```python
from build123d import *

# Parameters (mm, degrees)
BOSS_EXTRUDE1_DEPTH  = 90
BOSS_EXTRUDE2_DEPTH  = 70
BOSS_EXTRUDE4_DEPTH  = 10
SKETCH4_W            = 20
SKETCH4_H            = 40
BOSS_EXTRUDE6_DEPTH  = 20
CUT_EXTRUDE1_DEPTH   = 20
SKETCH9_W            = 20
SKETCH9_H            = 20
BOSS_EXTRUDE8_DEPTH  = 10
SKETCH10_W           = 20
SKETCH10_H           = 10
CUT_EXTRUDE2_DEPTH   = 10
BOSS_EXTRUDE9_START  = -10
BOSS_EXTRUDE9_DEPTH  = 20
SKETCH13_W           = 26.1880454
SKETCH13_H           = 20
BOSS_EXTRUDE13_DEPTH = 30
CUT_EXTRUDE3_DEPTH   = 10
BOSS_EXTRUDE14_DEPTH = 30
BOSS_EXTRUDE15_DEPTH = 30
BOSS_EXTRUDE16_DEPTH = 40
BOSS_EXTRUDE17_DEPTH = 40
BOSS_EXTRUDE18_DEPTH = 10


with BuildPart() as part:
    # Sketch1 → Boss-Extrude1 (new body)
    with BuildSketch(Plane.XY):
        Polygon((0, 0), (0, 30), (40, 30), (40, -30), (20, -30), (20, -20), align=None)
    extrude(amount=BOSS_EXTRUDE1_DEPTH)

    # Sketch2 → Boss-Extrude2 (add)
    with BuildSketch(Plane.XY.offset(70)):
        Polygon((0, 30), (-30, 30), (-30, 20), (-20, 20), (0, 0), align=None)
    extrude(amount=-BOSS_EXTRUDE2_DEPTH)

    # Sketch3 → Boss-Extrude4 (add)
    with BuildSketch(Plane(origin=(0, 30, 0), x_dir=(1, 0, 0), z_dir=(0, 1, 0))):
        Polygon((-30, -60), (-50, -40), (-30, -40), align=None)
    extrude(amount=-BOSS_EXTRUDE4_DEPTH)

    # Sketch4 → Boss-Extrude6 (add)
    with BuildSketch(Plane(origin=(0, 30, 0), x_dir=(1, 0, 0), z_dir=(0, 1, 0))):
        with Locations((-40, -20)):
            Rectangle(SKETCH4_W, SKETCH4_H)
    extrude(amount=-BOSS_EXTRUDE6_DEPTH)

    # Sketch6 → Cut-Extrude1 (cut)
    with BuildSketch(Plane.ZY.offset(50)):
        Polygon((40, 20), (30, 10), (40, 10), align=None)
    extrude(amount=-CUT_EXTRUDE1_DEPTH, mode=Mode.SUBTRACT)

    # Sketch9 → Boss-Extrude8 (add)
    with BuildSketch(Plane.XZ.offset(-10)):
        with Locations((-40, 10)):
            Rectangle(SKETCH9_W, SKETCH9_H)
    extrude(amount=BOSS_EXTRUDE8_DEPTH)

    # Sketch10 → Cut-Extrude2 (cut)
    with BuildSketch(Plane.ZY.offset(50)):
        with Locations((10, 5)):
            Rectangle(SKETCH10_W, SKETCH10_H)
    extrude(amount=-CUT_EXTRUDE2_DEPTH, mode=Mode.SUBTRACT)

    # Sketch11 → Boss-Extrude9 (add)
    with BuildSketch(Plane(origin=(-30, 0, 0), x_dir=(0, 0, -1), z_dir=(1, 0, 0)).offset(BOSS_EXTRUDE9_START)):
        Polygon((-20, 0), (-30, 10), (-20, 10), align=None)
    extrude(amount=BOSS_EXTRUDE9_DEPTH)

    # Sketch13 → Boss-Extrude13 (add)
    with BuildSketch(Plane(origin=(0, 0, 0), x_dir=(-1, 0, 0), z_dir=(0, 0, -1))):
        with Locations((16.9059773, 10)):
            Rectangle(SKETCH13_W, SKETCH13_H)
    extrude(amount=-BOSS_EXTRUDE13_DEPTH)

    # Sketch14 → Cut-Extrude3 (cut)
    with BuildSketch(Plane.ZY.offset(30)):
        Polygon((20, 0), (30, 10), (30, 0), align=None)
    extrude(amount=-CUT_EXTRUDE3_DEPTH, mode=Mode.SUBTRACT)

    # Sketch15 → Boss-Extrude14 (add)
    with BuildSketch(Plane.ZY.offset(50)):
        Polygon((30, 10), (30, 20), (40, 20), align=None)
    extrude(amount=-BOSS_EXTRUDE14_DEPTH)

    # Sketch16 → Boss-Extrude15 (add)
    with BuildSketch(Plane.XZ.offset(30)):
        Polygon((20, 0), (10, 0), (10, 40), (20, 60), align=None)
    extrude(amount=-BOSS_EXTRUDE15_DEPTH)

    # Sketch17 → Boss-Extrude16 (add)
    with BuildSketch(Plane(origin=(0, 0, 0), x_dir=(-1, 0, 0), z_dir=(0, 0, -1))):
        Polygon((-10, -30), (20, -10), (20, 0), (0, 0), (-10, -10), align=None)
    extrude(amount=-BOSS_EXTRUDE16_DEPTH)

    # Sketch18 → Boss-Extrude17 (add)
    with BuildSketch(Plane(origin=(0, 0, 0), x_dir=(-1, 0, 0), z_dir=(0, 0, -1))):
        Polygon((3.8119546, 3.8119546), (3.8119546, 0), (0, 0), align=None)
    extrude(amount=-BOSS_EXTRUDE17_DEPTH)

    # Sketch19 → Boss-Extrude18 (add)
    with BuildSketch(Plane.XY.offset(30)):
        Polygon((-3.8119546, 3.8119546), (-3.8119546, 0), (-20, 0), (-20, 20), align=None)
    extrude(amount=BOSS_EXTRUDE18_DEPTH)


solid = part.part
```
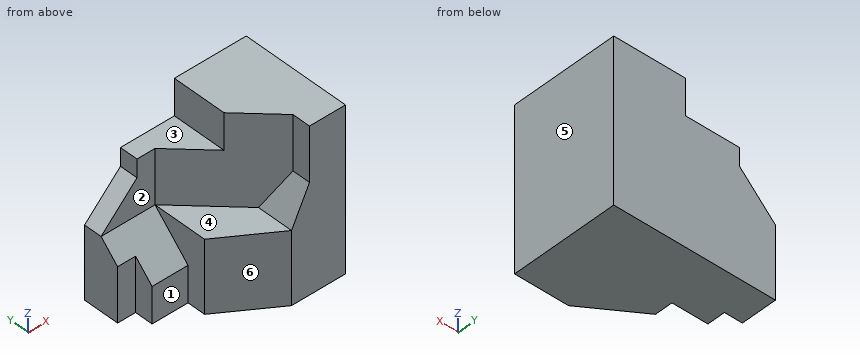
Input: part model. Units: mm. Frame: model coordinates. Face numbers are marked on the shaded views. A direction names the side the tool comes from. Give positions to 0.01 mm unless a question says otherwise; leave off trailing zeros. Write each loop counter-clockwise with the first axis right and the second up, starting at its lowest first coordinate (ties: lowest second). Pieces come first, ordered by that corner, then holes. Notation, with made-up numbers: (58.25, 57) - (101.25, 57) arc R12 ccw to (101.25, 76) - close; hole circle Ø4 at (70, -36.75). An arc over 180 degrees is marked (long way). Write item = value, one per line. Start each with the question number.
1) Pin query (flat end, axial travel): pin 1 (9 mm diameter, centred on x = -6, y = -7, fed in from +Z); pin 2 (3 mm diameter, centred on y = 25.5, z = 65, fed in from -X); pin 3 (5 mm diameter, centred on x = -47.5, z = 18, fed in from -Y). Return the tip coordinate at first contact, or that it passes through.
2) Cut plane D-D (y = 23.5). Return loops of the section in (x, z), and give its area (3 significant figures).
3) Cut plane B-B (y = -23.5). Return loops of the section in (x, z).
4) Material intervals for L1, parallel to X at y = 4, z = 81; L2, parallel to Y at x = -44, z = 41; L3, parallel to Z at x = -3.5, y = 16, sorted ascending. Write a range as [from, to].
5) Cut plane A-A (z = 53). Return loops of the section in (x, y).
6) Reachability of the marked faces 1, 2 and 3 from +Z, -Z, +X, -X, +Y, -Y: full face, straight path, thin tool, end or side. Return the list, or none.
7) Draft query along X for the marked faces 4, 5 and 6. Return one class per face: pulls with the +X half, pulls with the -X half, needs draft (parallel to the pull), parting line crosses it, or undercut.
8) Cut plane C-C (x = -26). Return loops of the section in (y, z).
Answers follow:
q1.pin_1 = 40
q1.pin_2 = -30
q1.pin_3 = 10
q2.outline = (-50, 0) - (40, 0) - (40, 90) - (0, 90) - (0, 70) - (-30, 70) - (-30, 60) - (-50, 40) - close
q2.area = 6,700 mm^2
q3.outline = (0.25, 0) - (40, 0) - (40, 90) - (20, 90) - (20, 60) - (10, 40) - (0.25, 40) - close
q4.L1 = [0, 40]
q4.L2 = [20, 30]
q4.L3 = [0, 70]
q5.outline = (-37, 20) - (-20, 20) - (16.5, -16.5) - (16.5, -30) - (40, -30) - (40, 30) - (-37, 30) - close
q6.face_1 = +Z, -Z, -X, -Y
q6.face_2 = +Z, -X, -Y
q6.face_3 = +Z, -X, +Y, -Y
q7.face_4 = needs draft
q7.face_5 = pulls with the +X half
q7.face_6 = pulls with the -X half
q8.outline = (0, 0) - (30, 0) - (30, 70) - (20, 70) - (20, 40) - (0, 20) - close
